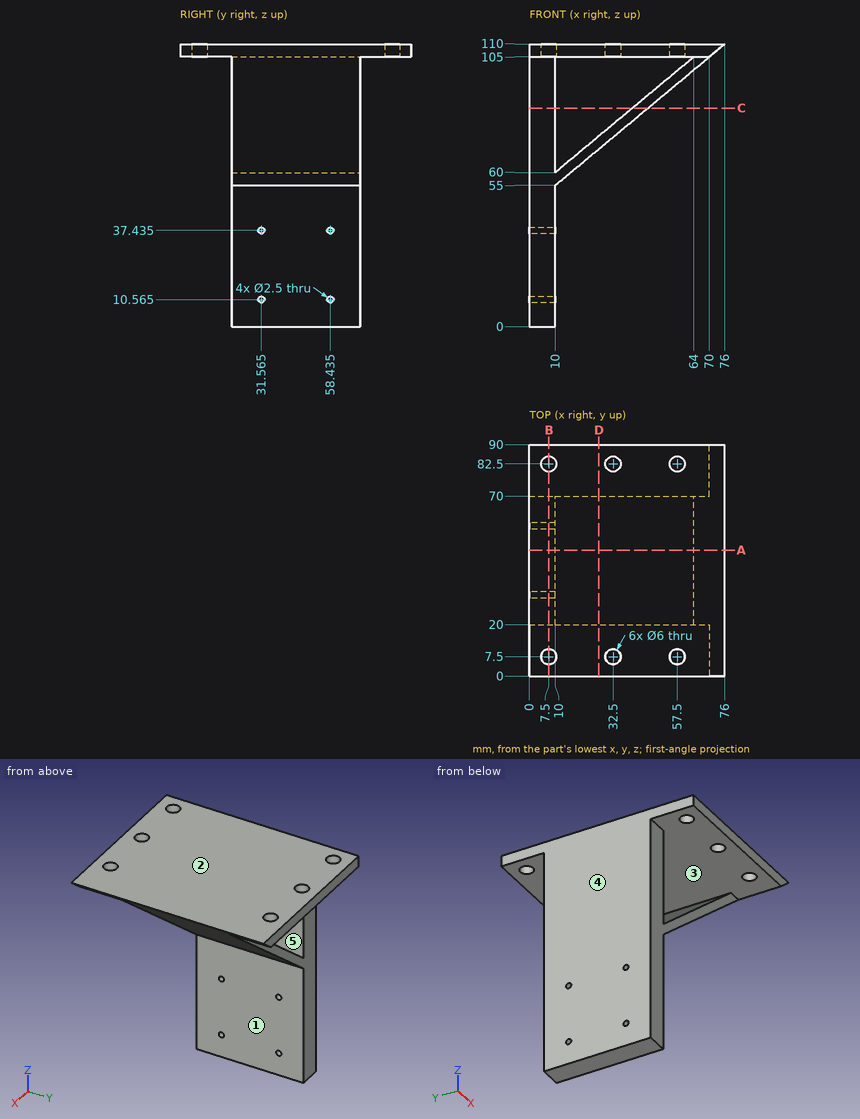
Check sheet for the drawn part. Datum: minimum x, y, z corner. Units: mm. A direction names the side the tool comes from. Give positions to 0.01 mm unless a question says otherwise; leave off trailing zeros. Order: outer loops, then holes, each group sorted by start corner. A loop starts at its lowest first (then second) coordinate and runs counter-clockwise, first axis right, second up.
1. Sectioned sample at A-A (y = 49). Record the boundary of the cut face in (x, z).
Completed:
outline: (0, 0) - (10, 0) - (10, 55) - (76, 110) - (0, 110) - close; hole (10, 60) - (64, 105) - (10, 105) - close
2. Sectioned sample at B-B (x = 7.5). Record the boundary of the cut face in (y, z) (3 decimals).
Completed:
outline: (0, 105) - (4.5, 105) - (4.5, 110) - (0, 110) - close; (10.5, 105) - (20, 105) - (20, 0) - (70, 0) - (70, 105) - (79.5, 105) - (79.5, 110) - (10.5, 110) - close; (85.5, 105) - (90, 105) - (90, 110) - (85.5, 110) - close; hole circle Ø2.5 at (31.565, 10.565); hole circle Ø2.5 at (31.565, 37.435); hole circle Ø2.5 at (58.435, 10.565); hole circle Ø2.5 at (58.435, 37.435)
3. Access from +Z, -Z, +X, -X, +Y, -Y to the whole of each face (thin tool, end or side, straight path). Record for the marked faces 4 and 5.
Completed:
face 4: +Z, -Z, -X, +Y, -Y
face 5: +Y, -Y
4. Scan lines: line 1 (Y direction, x = 57.5, z = 107.7); line 2 (X direction, y = 54, z = 24.5); line 3 (Z direction, x = 54.5, y = 80). Record each from-to range of solid material in increasing order.
Completed:
line 1: y = 0 to 4.5, 10.5 to 79.5, 85.5 to 90
line 2: x = 0 to 10
line 3: z = 105 to 110
5. Sectioned sample at D-D (x = 27). Record the boundary of the cut face in (y, z).
Completed:
outline: (0, 105) - (90, 105) - (90, 110) - (0, 110) - close; (20, 69.17) - (70, 69.17) - (70, 74.17) - (20, 74.17) - close
6. Sectioned sample at C-C (z = 85). Record the boundary of the cut face in (x, y), then the cut area to 3 significant figures.
Completed:
outline: (0, 20) - (10, 20) - (10, 70) - (0, 70) - close; (40, 20) - (46, 20) - (46, 70) - (40, 70) - close
area: 800 mm2
7. Draft check along Z on the marked faces 1, 2 and 3. Enter one of: pulls with the +Z half, pulls with the -Z half, needs draft (parallel to the pull), parting line crosses it, or undercut.
Completed:
face 1: needs draft
face 2: pulls with the +Z half
face 3: undercut
8. Depth check by flat-ended pin: pin 1 (22.5 mm diameter, centred on y = 35, z = 83, fed in from +X); pin 2 (7 mm diameter, centred on x = 32.5, y = 7.5, fed in from -Z); pin 3 (15 mm diameter, centred on y = 44.5, z = 37.5, fed in from +X). Enter the tip coordinate at first touch or a pass-through.
Completed:
pin 1: stops at x = 57.1
pin 2: stops at z = 105
pin 3: stops at x = 10
